Source: CAD feature listing. Evaluate the final solid. Frame: model axes, mm. Face numbers are marked on the shaded views. A direction names the side the tool comes from. Coordinates: 2 decimals unless noted, no trailing zeros. Order: outer loops, then holes, each group sorted by start corner. A loop starts at its lowest first (then second) coordinate and runs counter-clockwise, first axis right, second up.
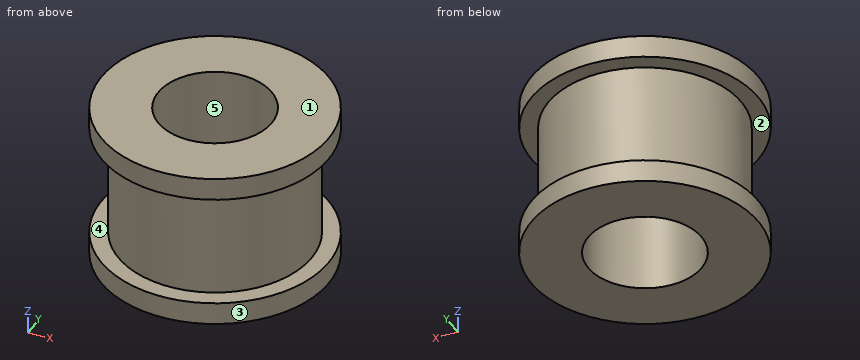
```python
from build123d import *

# Parameters (mm, degrees)
F0_R          = 10
F1_DEPTH      = 2
F2_R          = 8.5
F3_DEPTH      = 10
F4_R          = 10
F5_DEPTH      = 2
F6_R          = 5
F7_DEPTH      = 20
F7_DEPTH_BACK = 6


with BuildPart() as f1:
    # F0 (on Top) → F1 (new body)
    with BuildSketch(Plane.XY):
        Circle(F0_R)
    extrude(amount=F1_DEPTH)

    # F2 (on face) → F3 (join)
    with BuildSketch(Plane.XY.offset(2)):
        Circle(F2_R)
    extrude(amount=F3_DEPTH)

    # F4 (on face) → F5 (join)
    with BuildSketch(Plane.XY.offset(12)):
        Circle(F4_R)
    extrude(amount=F5_DEPTH)

    # F6 (on face) → F7 (cut, two sides)
    with BuildSketch(Plane.XY.offset(14)) as f7_sk:
        Circle(F6_R)
    extrude(amount=-F7_DEPTH, mode=Mode.SUBTRACT)
    extrude(f7_sk.sketch, amount=-F7_DEPTH_BACK, mode=Mode.SUBTRACT)


solid = f1.part
```
Q1. Set-up query: the marked faces 1 and 2. Return all of +Z, -Z, +X, -X, +Y, -Y with unobstructed straight access to the full face (end or side cutting, diameter ignored); none if empty.
Solutions:
face 1: +Z, +X, -X, +Y, -Y
face 2: none
Q2. Section query C-C on z = 10.25. Output: boundary loops of the cut face in (x, y).
Solutions:
outline: circle Ø17 at (0, 0); hole circle Ø10 at (0, 0)
Q3. Pin query (flat end, axial travel): P1, Ø8, axis at x = 0, y = 0, coming from the +Z side; P2, Ø5, axis at y = 0.5, z = 5, coming from the +X side; P3, Ø2, axis at x = -2, z = 5, coming from the +Y side; P4, Ø1, axis at y = -3.5, z = 8.5, coming from the +X side. Return the tip coordinate at first contact, or that it passes through.
Solutions:
P1: passes through
P2: stops at x = 8.5
P3: stops at y = 8.44
P4: stops at x = 7.95
Q4. Pull-direction query (X, two-part tool) for the marked faces 3, 4 and 5; classes: pulls with the +X half, pulls with the -X half, needs draft (parallel to the pull), parting line crosses it, or undercut.
Solutions:
face 3: parting line crosses it
face 4: needs draft
face 5: undercut
Q5. Section query A-A on y = 0. Output: boundary loops of the cut face in (x, z), plus the area to 3 significant figures.
Solutions:
outline: (-10, 0) - (-5, 0) - (-5, 14) - (-10, 14) - (-10, 12) - (-8.5, 12) - (-8.5, 2) - (-10, 2) - close; (5, 0) - (10, 0) - (10, 2) - (8.5, 2) - (8.5, 12) - (10, 12) - (10, 14) - (5, 14) - close
area: 110 mm2
Q6. Material intervals for line 1 along Y through (x, z) = (0, 9.75); line 2 along Z through (x, y) = (8.5, 4.25); line 3 along Y through (x, z) = (0.25, 12.5), sorted ascending.
Solutions:
line 1: y = -8.5 to -5, 5 to 8.5
line 2: z = 0 to 2, 12 to 14
line 3: y = -10 to -4.99, 4.99 to 10
Q7. Section query D-D on y = 7.75. Output: boundary loops of the cut face in (x, z), plus the area to 3 significant figures.
Solutions:
outline: (-6.32, 0) - (6.32, 0) - (6.32, 2) - (3.49, 2) - (3.49, 12) - (6.32, 12) - (6.32, 14) - (-6.32, 14) - (-6.32, 12) - (-3.49, 12) - (-3.49, 2) - (-6.32, 2) - close
area: 120 mm2
